from build123d import *

# Parameters (mm, degrees)
SKETCH1_W                 = 76.21
SKETCH1_H                 = 51.5
BOSS_EXTRUDE1_DEPTH       = 25
SHELL1_T                  = -2
CUT_EXTRUDE1_DEPTH        = 53.345520582
SKETCH4_W                 = 43.999864015
SKETCH4_H                 = 51.5
SKETCH4_W_2               = 39.690462938
SKETCH4_H_2               = 47.5
BOSS_EXTRUDE2_DEPTH       = 10
BOSS_EXTRUDE3_REACH       = 75.765
FILLET1_R                 = 0.5
FILLET3_R                 = 6
FILLET1_OF_MIRROR3_R      = 0.5
FILLET3_OF_MIRROR3_R      = 6
CUT_EXTRUDE2_DEPTH        = 74.765193194
BOSS_EXTRUDE4_REACH       = 75.765
SKETCH7_W                 = 24.449300912
SKETCH7_H                 = 1.5
CUT_EXTRUDE3_REACH        = 79.215
LPATTERN1_COUNT           = 2
LPATTERN1_PITCH           = 8
SKETCH9_R                 = 2
SKETCH9_R_2               = 1.5
BOSS_EXTRUDE5_DEPTH       = 5
SKETCH10_W                = 4
SKETCH10_H                = 4
BOSS_EXTRUDE6_DEPTH       = 7
BOSS_EXTRUDE7_DEPTH       = 10.35
SKETCH12_R                = 2
BOSS_EXTRUDE8_DEPTH       = 10
F_1_5MM_DOWEL_HOLE1_D     = 1.5
F_1_5MM_DOWEL_HOLE1_DEPTH = 5
F_1_5MM_DOWEL_HOLE1_TIP   = 0.450645464
FILLET5_R                 = 1
SKETCH15_W                = 19
SKETCH15_H                = 51.5
SKETCH15_W_2              = 15
SKETCH15_H_2              = 47.5
BOSS_EXTRUDE9_DEPTH       = 10
CUT_EXTRUDE4_REACH        = 91.835
SKETCH16_W                = 15
SKETCH16_H                = 47.5
BOSS_EXTRUDE10_REACH      = 91.93
SKETCH19_W                = 10
SKETCH19_H                = 7.5


with BuildPart() as part:
    # Sketch1 → Boss-Extrude1 (new, symmetric)
    with BuildSketch(Plane.XY):
        Rectangle(SKETCH1_W, SKETCH1_H)
    extrude(amount=BOSS_EXTRUDE1_DEPTH, both=True)

    # Shell1
    shell1_openings = [part.faces().sort_by_distance(p)[0] for p in [
        (0, 0, -25),
    ]]
    offset(amount=SHELL1_T, openings=shell1_openings, kind=Kind.INTERSECTION)

    # Sketch3 → Cut-Extrude1 (cut, symmetric)
    with BuildSketch(Plane(origin=(0, 0, 0), x_dir=(1, 0, 0), z_dir=(0, 1, 0))):
        Polygon((0, -25), (-38.105, -3.000067993), (-38.105, -25), align=None)
    cut_extrude1 = extrude(amount=CUT_EXTRUDE1_DEPTH, both=True, mode=Mode.SUBTRACT)

    # Mirror1: Cut-Extrude1 across plane
    add(cut_extrude1.mirror(Plane(origin=(0, 0, 0), x_dir=(0, 0, 1), z_dir=(1, 0, 0))), mode=Mode.SUBTRACT)

    # Sketch4 → Boss-Extrude2 (add)
    with BuildSketch(Plane(origin=(-10.825317547, 0, 18.75), x_dir=(0.8660254037844363, 0, 0.5000000000000042), z_dir=(-0.5000000000000041, 0, 0.8660254037844362))):
        with Locations((-9.499932008, 0)):
            Rectangle(SKETCH4_W, SKETCH4_H)
        with Locations((-9.345231469, 0)):
            Rectangle(SKETCH4_W_2, SKETCH4_H_2, mode=Mode.SUBTRACT)
    boss_extrude2 = extrude(amount=BOSS_EXTRUDE2_DEPTH)

    # Mirror2: Boss-Extrude2 across plane
    add(boss_extrude2.mirror(Plane(origin=(0, 0, 0), x_dir=(0, 0, 1), z_dir=(1, 0, 0))))

    # Sketch5 → Boss-Extrude3 (add, up to next)
    with BuildSketch(Plane(origin=(0, -23.75, 0), x_dir=(1, 0, 0), z_dir=(0, 1, 0)), mode=Mode.PRIVATE) as boss_extrude3_sk1:
        Polygon((-22, 19.866199846), (-36.105, 25), (-36.105, 23.5), (-23.5, 18.912155197), (-23.5, -4.154768531), (-22, -4.154768531), align=None)
    boss_extrude3_tool1 = extrude(boss_extrude3_sk1.sketch, amount=BOSS_EXTRUDE3_REACH, mode=Mode.PRIVATE) - part.part
    boss_extrude3 = boss_extrude3_tool1.solids().sort_by_distance((-29.163272, -23.75, -22.128757))[0]
    add(boss_extrude3)

    # Fillet1
    fillet1_edges = [part.edges().sort_by_distance(p)[0] for p in [
        (-22, 0, 4.154768531),
        (-23.5, 0, 4.154768531),
    ]]
    fillet(fillet1_edges, radius=FILLET1_R)

    # Fillet3
    fillet3_edges = [part.edges().sort_by_distance(p)[0] for p in [
        (-22, 0, -19.866199846),
        (-23.5, 0, -18.912155197),
    ]]
    fillet(fillet3_edges, radius=FILLET3_R)

    # Mirror3: Boss-Extrude3 across plane
    add(boss_extrude3.mirror(Plane(origin=(0, 0, 0), x_dir=(0, 0, 1), z_dir=(1, 0, 0))))

    # Fillet1 of Mirror3
    fillet1_of_mirror3_edges = [part.edges().sort_by_distance(p)[0] for p in [
        (22, 0, 4.154768531),
        (23.5, 0, 4.154768531),
    ]]
    fillet(fillet1_of_mirror3_edges, radius=FILLET1_OF_MIRROR3_R)

    # Fillet3 of Mirror3
    fillet3_of_mirror3_edges = [part.edges().sort_by_distance(p)[0] for p in [
        (22, 0, -19.866199846),
        (23.5, 0, -18.912155197),
    ]]
    fillet(fillet3_of_mirror3_edges, radius=FILLET3_OF_MIRROR3_R)

    # Sketch6 → Cut-Extrude2 (cut, through all)
    with BuildSketch(Plane(origin=(0, -23.75, 0), x_dir=(1, 0, 0), z_dir=(0, 1, 0))):
        Polygon((-28.344300912, 25), (11.655699088, 25), (11.655699088, 15), (8.655699088, 15), (8.655699088, -2), (-16.344300912, -2), (-16.344300912, 15), (-28.344300912, 15), align=None)
    extrude(amount=-CUT_EXTRUDE2_DEPTH, mode=Mode.SUBTRACT)

    # Sketch7 → Boss-Extrude4 (add, up to next)
    with BuildSketch(Plane(origin=(0, -23.75, 0), x_dir=(1, 0, 0), z_dir=(0, 1, 0)), mode=Mode.PRIVATE) as boss_extrude4_sk1:
        with Locations((23.880349544, 24.25)):
            Rectangle(SKETCH7_W, SKETCH7_H)
    boss_extrude4_tool1 = extrude(boss_extrude4_sk1.sketch, amount=BOSS_EXTRUDE4_REACH, mode=Mode.PRIVATE) - part.part
    add(boss_extrude4_tool1.solids().sort_by_distance((23.88035, -23.75, -24.25))[0])

    # Sketch8 → Cut-Extrude3 (cut, up to next)
    with BuildSketch(Plane(origin=(0, 0, -25), x_dir=(-1, 0, 0), z_dir=(0, 0, -1)), mode=Mode.PRIVATE) as cut_extrude3_sk1:
        with BuildLine():
            Line((-14.655699088, 19), (-14.655699088, -21))
            ThreePointArc((-14.655699088, -21), (-16.655699088, -23), (-18.655699088, -21))
            Line((-18.655699088, -21), (-18.655699088, 19))
            ThreePointArc((-18.655699088, 19), (-16.655699088, 21), (-14.655699088, 19))
        make_face()
    cut_extrude3_tool1 = extrude(cut_extrude3_sk1.sketch, amount=-CUT_EXTRUDE3_REACH, mode=Mode.PRIVATE) & part.part
    cut_extrude3 = cut_extrude3_tool1.solids().sort_by_distance((16.655699, -1, -25))[0]
    add(cut_extrude3, mode=Mode.SUBTRACT)

    # LPattern1: Cut-Extrude3 ×2
    with Locations(*[(i * LPATTERN1_PITCH, 0, 0) for i in range(1, LPATTERN1_COUNT)]):
        add(cut_extrude3, mode=Mode.SUBTRACT)



with BuildPart() as body_2:
    # Sketch9 → Boss-Extrude5 (new body)
    with BuildSketch(Plane(origin=(0, 0, -25), x_dir=(-1, 0, 0), z_dir=(0, 0, -1))):
        with Locations((21.844300912, 11.4)):
            Circle(SKETCH9_R)
        with Locations((21.844300912, 11.4)):
            Circle(SKETCH9_R_2, mode=Mode.SUBTRACT)
    extrude(amount=-BOSS_EXTRUDE5_DEPTH)

    # Sketch10 → Boss-Extrude6 (add)
    with BuildSketch(Plane.XY.offset(-20)):
        with Locations((-21.844300912, 11.4)):
            Rectangle(SKETCH10_W, SKETCH10_H)
    extrude(amount=BOSS_EXTRUDE6_DEPTH)


with BuildPart() as part_1:
    add(part.part)

    add(body_2.part)  # Boss-Extrude7 merges body 2
    # Sketch11 → Boss-Extrude7 (add)
    with BuildSketch(Plane(origin=(0, 13.4, 0), x_dir=(1, 0, 0), z_dir=(0, 1, 0))):
        Polygon((-19.844300912, 20), (-21.844300912, 20), (-23.844300912, 20), (-23.844300912, 13), (-19.844300912, 13), align=None)
    extrude(amount=BOSS_EXTRUDE7_DEPTH)

    # Sketch12 → Boss-Extrude8 (add)
    with BuildSketch(Plane(origin=(0, 0, -25), x_dir=(-1, 0, 0), z_dir=(0, 0, -1))):
        with Locations((39.344300912, -7.5)):
            Circle(SKETCH12_R)
    extrude(amount=-BOSS_EXTRUDE8_DEPTH)

    # Ø1.5mm Dowel Hole1
    with Locations(Plane(origin=(0, 0, -25), x_dir=(-1, 0, 0), z_dir=(0, 0, -1))):
        with Locations((39.344300912, -7.5)):
            Hole(F_1_5MM_DOWEL_HOLE1_D / 2, depth=F_1_5MM_DOWEL_HOLE1_DEPTH)
            with Locations((0, 0, -(F_1_5MM_DOWEL_HOLE1_DEPTH + F_1_5MM_DOWEL_HOLE1_TIP / 2))):  # 118° drill point
                Cone(0, F_1_5MM_DOWEL_HOLE1_D / 2, F_1_5MM_DOWEL_HOLE1_TIP, mode=Mode.SUBTRACT)

    # Fillet5
    fillet5_edges = [part_1.edges().sort_by_distance(p)[0] for p in [
        (0, 0, 25),
    ]]
    fillet(fillet5_edges, radius=FILLET5_R)

    # Sketch15 → Boss-Extrude9 (add)
    with BuildSketch(Plane.ZY.offset(-36.105)):
        with Locations((-15.5, 0)):
            Rectangle(SKETCH15_W, SKETCH15_H)
        with Locations((-15.5, 0)):
            Rectangle(SKETCH15_W_2, SKETCH15_H_2, mode=Mode.SUBTRACT)
    boss_extrude9 = extrude(amount=-BOSS_EXTRUDE9_DEPTH)

    # Sketch16 → Cut-Extrude4 (cut, up to next)
    with BuildSketch(Plane.ZY.offset(-36.105), mode=Mode.PRIVATE) as cut_extrude4_sk1:
        with Locations((-15.5, 0)):
            Rectangle(SKETCH16_W, SKETCH16_H)
    cut_extrude4_tool1 = extrude(cut_extrude4_sk1.sketch, amount=-CUT_EXTRUDE4_REACH, mode=Mode.PRIVATE) & part_1.part
    cut_extrude4 = cut_extrude4_tool1.solids().sort_by_distance((36.105, 0, -15.5))[0]
    add(cut_extrude4, mode=Mode.SUBTRACT)

    # Mirror4: Boss-Extrude9, Cut-Extrude4 mirrored; each copy of Cut-Extrude4 runs up to whatever stops it at its own place
    mirror4_before = part_1.part  # the part as the pattern finds it: every copy runs up to it
    add(boss_extrude9.mirror(Plane(origin=(0, 0, 0), x_dir=(0, 0, 1), z_dir=(1, 0, 0))))
    mirror4_cut_extrude4_long = extrude(cut_extrude4_sk1.sketch, amount=-CUT_EXTRUDE4_REACH, mode=Mode.PRIVATE)
    mirror4_cut_extrude4_tool = mirror4_cut_extrude4_long.mirror(Plane(origin=(0, 0, 0), x_dir=(0, 0, 1), z_dir=(1, 0, 0))) & mirror4_before
    add(mirror4_cut_extrude4_tool.solids().sort_by_distance((-36.105, 0, -15.5))[0], mode=Mode.SUBTRACT)

    # Sketch19 → Boss-Extrude10 (add, up to next)
    with BuildSketch(Plane(origin=(-25.279682453, 0, -14.595231469), x_dir=(0.5000000000000041, 0, -0.8660254037844364), z_dir=(0.8660254037844364, 0, 0.5000000000000041)), mode=Mode.PRIVATE) as boss_extrude10_sk1:
        with Locations((-26.650635095, 20)):
            Rectangle(SKETCH19_W, SKETCH19_H)
    boss_extrude10_tool1 = extrude(boss_extrude10_sk1.sketch, amount=BOSS_EXTRUDE10_REACH, mode=Mode.PRIVATE) - part_1.part
    boss_extrude10 = boss_extrude10_tool1.solids().sort_by_distance((-38.605, 20, 8.484896))[0]
    add(boss_extrude10)

    # Mirror5: Boss-Extrude10 across plane
    add(boss_extrude10.mirror(Plane(origin=(0, 0, 0), x_dir=(0, 0, 1), z_dir=(1, 0, 0))))


solid = part_1.part
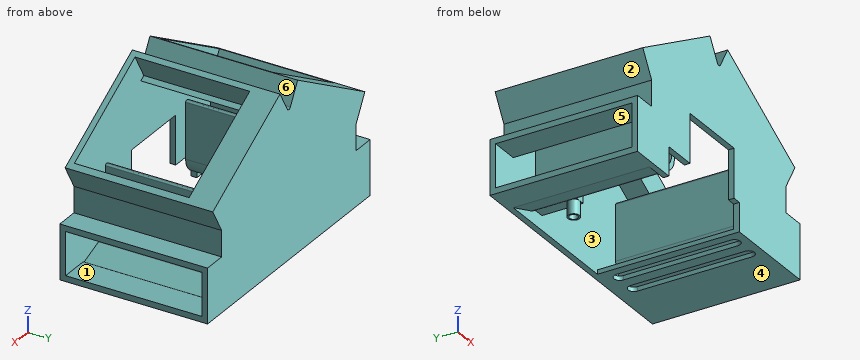
Check sheet for the modelled part. Datum: model origin and axes. Units: mm. Face numbers are marked on the shaded views. A direction names the side the tool comes from. Round coordinates to 2 decimals unless told otherwise and drop trailing zeros. Loops run counter-clockwise (first coordinate to the right, second up) from the corner with the lowest first, then second, coordinate; pieces in that order, holes last.
1. Mould release check, pull along Z, two halves, no side actions. Record for the marked faces 4, 5 and 6: released by +Z, released by -Z, zero draft, split by the parting line, or undercut.
2. Sectioned sample at B-B on z = 18. Record the boundary of the cut face in (x, y).
3. Scan lines: probe 1 along X at (y, z) = (-16, -5) (3 decimals); probe 2 along Y at (x, z) = (24, 5); probe 3 along X at (y, z) = (-1, -14). Record each from-to range of solid material in increasing order.
4. Set-up check for the marked faces 1, 2 and 3: record each of +Z, -Z, +X, -X, +Y, -Y from which the full face is reachable in a straight line by a thin tool's end or side.
5. Sectioned sample at A-A on x = -11.5. Record the boundary of the cut face in (y, z), and give its area (3 significant figures).
6. Sectioned sample at C-C on z = 10.5. Record the boundary of the cut face in (x, y).
7. Gauge pin test, flat ends, axial feed: pin 1 Ø5 at (y, z) = (7, -16) entering from -X; pin 2 Ø1.5 at (y, z) = (-0.5, 14.5) entering from -X; pin 3 Ø3 at (x, y) = (2.5, 13.5) entering from -Z; pin 4 Ø2 at (y, z) = (-10.5, -1) entering from +X (3 decimals). Record the tip position at first contact, or that the pin passes through.
8. Sectioned sample at D-D on y = -20. Give the number of separate pieces and of enclosed holes in the cut face, and give its area (3 significant figures).
Recorded:
1. face 4: released by -Z
1. face 5: undercut
1. face 6: released by +Z
2. outline: (-32.12, -25.75) - (32.12, -25.75) - (32.12, -23.75) - (-32.12, -23.75) - close; (-32.12, 16.25) - (-12.12, 16.25) - (-12.12, 23.75) - (12.12, 23.75) - (12.12, 16.25) - (32.12, 16.25) - (32.12, 25.75) - (-32.12, 25.75) - close
3. probe 1: x = -38.105 to -36.105, -23.5 to -22, 22 to 23.5, 36.105 to 38.105
3. probe 2: y = -25.75 to -23.75, 23.75 to 25.75
3. probe 3: x = -23.5 to -22, 22 to 23.5
4. face 1: +X
4. face 2: -X, +Y, -Y
4. face 3: none
5. outline: (-25.75, 2) - (-23.75, 2) - (-23.75, 29.91) - (-25.75, 29.91) - close; (16.25, 18.36) - (23.75, 18.36) - (23.75, -25) - (25.75, -25) - (25.75, 29.91) - (16.25, 29.91) - close
5. area: 252 mm2
6. outline: (-42.44, -25.75) - (42.44, -25.75) - (42.44, 25.75) - (-42.44, 25.75) - close; hole (-39.77, -23.75) - (39.77, -23.75) - (39.77, 16.25) - (25.11, 16.25) - (25.11, 23.75) - (-25.11, 23.75) - (-25.11, 16.25) - (-39.77, 16.25) - close
7. pin 1: stops at x = -24.85
7. pin 2: passes through
7. pin 3: stops at z = 23
7. pin 4: stops at x = 38.105
8. separate pieces: 7
8. enclosed holes: 0
8. area: 344 mm2
